The model under review builds one solid part; all positions refer to its coordinate system, in mm. A direction names the side the tool comes from. Round coordinates to 2 decimals unless told otherwise and drop trailing zeros. Return JSON: item names as keys, results as strings. Group by question number.
```python
from build123d import *

# Parameters (mm, degrees)
SKETCH3_W           = 30
SKETCH3_H           = 5
SKETCH3_W_2         = 5
SKETCH3_H_2         = 30
BOSS_EXTRUDE2_DEPTH = 25
CUT_EXTRUDE2_DEPTH  = 35.003676272
BOSS_EXTRUDE3_DEPTH = 5
SKETCH9_W           = 12.5
SKETCH9_H           = 5
CUT_EXTRUDE3_DEPTH  = 50.460787365
CIRPATTERN9_COUNT   = 4
SKETCH11_W          = 30
SKETCH11_H          = 25
BOSS_EXTRUDE5_DEPTH = 2.5
FILLET1_R           = 3


with BuildPart() as part:
    # Sketch3 → Boss-Extrude2 (new body)
    with BuildSketch(Plane(origin=(0, 0, 0), x_dir=(1, 0, 0), z_dir=(0, 1, 0))):
        Rectangle(SKETCH3_W, SKETCH3_H)
        Rectangle(SKETCH3_W_2, SKETCH3_H_2)
    extrude(amount=BOSS_EXTRUDE2_DEPTH)

    # Sketch4 → Cut-Extrude2 (cut, symmetric)
    with BuildSketch(Plane(origin=(2.5, 0, 0), x_dir=(0, 0, -1), z_dir=(1, 0, 0))):
        with BuildLine():
            Line((-15, 25), (-15, 17.357377201))
            add(Edge.make_bspline(
                [(-15, 17.357377201), (-12.472140197, 21.356054213), (-10.128526377, 24.727998236), (-4.127581327, 25)],
                knots=[0.577139171, 0.577139171, 0.577139171, 0.577139171, 0.966590179, 0.966590179, 0.966590179, 0.966590179], degree=3))
            Line((-4.127581327, 25), (-15, 25))
        make_face()
    cut_extrude2 = extrude(amount=CUT_EXTRUDE2_DEPTH, both=True, mode=Mode.SUBTRACT)

    # Sketch5 → Boss-Extrude3 (add)
    with BuildSketch(Plane(origin=(2.5, 0, 0), x_dir=(0, 0, -1), z_dir=(1, 0, 0))):
        with BuildLine():
            Line((-39.95459265, 0), (-15, 0))
            Line((-15, 0), (-15, 17.357377201))
            add(Edge.make_bspline(
                [(-39.95459265, 3.5), (-22.896848779, 4.129478661), (-18.746111538, 11.431617363), (-15, 17.357377201)],
                knots=[0, 0, 0, 0, 0.577139171, 0.577139171, 0.577139171, 0.577139171], degree=3))
            Line((-39.95459265, 3.5), (-39.95459265, 0))
        make_face()
    boss_extrude3 = extrude(amount=-BOSS_EXTRUDE3_DEPTH)

    # Mirror1: Boss-Extrude3 across plane
    add(boss_extrude3.mirror(Plane.XY))

    # Mirror2: Cut-Extrude2 across plane
    add(cut_extrude2.mirror(Plane.XY), mode=Mode.SUBTRACT)

    # Sketch9 → Cut-Extrude3 (cut, through all)
    with BuildSketch(Plane(origin=(0, 25, 0), x_dir=(1, 0, 0), z_dir=(0, 1, 0))):
        with Locations((-8.75, 0)):
            Rectangle(SKETCH9_W, SKETCH9_H)
        with Locations((8.75, 0)):
            Rectangle(SKETCH9_W, SKETCH9_H)
    extrude(amount=-CUT_EXTRUDE3_DEPTH, mode=Mode.SUBTRACT)


with BuildPart() as cirpattern9_1:
    # CirPattern9: pattern copy
    add(part.part.rotate(Axis((0, 0, 0), (0, 1, 0)), 1 * 360 / CIRPATTERN9_COUNT))


with BuildPart() as cirpattern9_2:
    # CirPattern9: pattern copy
    add(part.part.rotate(Axis((0, 0, 0), (0, 1, 0)), 2 * 360 / CIRPATTERN9_COUNT))


with BuildPart() as cirpattern9_3:
    # CirPattern9: pattern copy
    add(part.part.rotate(Axis((0, 0, 0), (0, 1, 0)), 3 * 360 / CIRPATTERN9_COUNT))


with BuildPart() as part_1:
    add(part.part)

    add(cirpattern9_1.part)  # Boss-Extrude5 merges CirPattern9_1

    add(cirpattern9_2.part)  # Boss-Extrude5 merges CirPattern9_2

    add(cirpattern9_3.part)  # Boss-Extrude5 merges CirPattern9_3
    # Sketch11 → Boss-Extrude5 (add, symmetric)
    with BuildSketch(Plane(origin=(0, 0, 0), x_dir=(0.7071067811865489, 0, 0.7071067811865462), z_dir=(-0.7071067811865462, 0, 0.7071067811865489))):
        with Locations((0, 12.5)):
            Rectangle(SKETCH11_W, SKETCH11_H)
    extrude(amount=BOSS_EXTRUDE5_DEPTH, both=True)

    # Fillet1
    fillet1_edges = [part_1.edges().sort_by_distance(p)[0] for p in [
        (0, 3.5, 39.95459265),
        (0, 3.5, -39.95459265),
        (39.95459265, 3.5, 0),
        (-39.95459265, 3.5, 0),
    ]]
    fillet(fillet1_edges, radius=FILLET1_R)


solid = part_1.part
```
1. Wall thickness on line 1 (X direction, y = 9.25, z = -13.5); line 2 (X direction, y = 2.5, z = 11.5); line 3 (Z direction, x = 7, y = 9.5): over which ranges is each line inside the solid? List them lowest first.
2. Draft analysis for pull direction Z (two halves, no side actions). For faces 1 (the face through (10.582, 12.325, 10.631)), 2 (the face through (2.5, 7, 15)), 3 (the face through (9.11, 12.675, 5.574)), 4 (the face through (-16, 10, -2.5)), state which applies: pulls with the +Z half, pulls with the -Z half, needs draft (parallel to the pull), parting line crosses it, or undercut.
3. For P1, Ø7.5, axis at x = -16.5, y = 8, coming from the -Z side; P2, Ø6, axis at y = 15.5, z = 17.5, coming from the -X side; P3, Ø12.5, axis at y = 7.5, z = -25, coming from the +X side, all flat-tipped, find the tip position at first contact; note any pin that passes through.
4. Tool access review of faces 5 (the face through (0, 25, 0)), 6 (the face through (-2.5, 10, 13)), 7 (the face through (13, 10, -2.5)), 8 (the face through (-10.631, 12.325, -10.582)), 9 (the face through (-2.5, 7, -15)): name each direction out of +Z, -Z, +X, -X, +Y, -Y from which nothing blocks a thin tool from reaching the whole face with its end or side.
Check sheet entries:
{
 "1": {"line 1": "x = -2.5 to 2.5", "line 2": "x = -2.5 to 2.5, 7.96 to 9.71", "line 3": "z = -2.5 to 2.5, 3.46 to 10.54"},
 "2": {"face 1": "pulls with the +Z half", "face 2": "needs draft", "face 3": "undercut", "face 4": "undercut"},
 "3": {"P1": "stops at z = -2.5", "P2": "stops at x = -2.5", "P3": "stops at x = 2.5"},
 "4": {"face 5": "+Z, -Z, +X, -X, +Y", "face 6": "+Z, -X, +Y, -Y", "face 7": "-Z, +X, +Y, -Y", "face 8": "-Z, -X, +Y, -Y", "face 9": "-Z, +Y, -Y"}
}
